Could you check a few things on this model? Use its own coordinates, in mm. A direction names the side the tool comes from. Give positions to 0.01 mm unless a question says otherwise; leave off trailing zeros. Loops run counter-clockwise (first coordinate to the right, second up) from the corner with the lowest first, then second, coordinate; pieces in that order, holes last.
1. Imagine slicing it at C-C (z = 11). List the corners of the cut face in (x, y) for me.
2. Imagine slicing it at B-B (x = 64.5). List the corners of the cut face in (y, z) for me (3 decimals), plus the area to 3 significant figures.
3. For faces 1 (the flat face through (-4, 5.334, 0)), 2 (the flat face through (47, -3.175, 0)), 3 (the cylindrical face through (8.82, 13.08, -2.9)), 4 (the flat face through (-1, 3.175, 22)), which set-ups out of +Z, -Z, +X, -X, +Y, -Y let a thin tool reach every point of the face, with its end or its side?
4. For P1, Ø4.5, axis at x = 59.5, z = 0, coming from the +Y side (3 decimals); P2, Ø6, axis at y = 13, z = -2.5, coming from the -X side; P3, Ø0.9, axis at y = -0.5, z = 22.5, coming from the -X side, each with a flat end and sliding along its axis, tell me the tip position at first contact or that it passes through.
5. I need wall thicknesses on line 1 along Y through (x, z) = (12.5, 0); line 2 along X through (y, z) = (0, -9); line 3 along Y through (x, z) = (41, 7) (3 decimals). Which ranges of each line are inside material? Lowest first, please.
6. Thinking about a two-plate mould opening in Z: for faces 5 (the cylindrical face through (-3.78, -0.07, 24.51)), 6 (the flat face through (47, 3.175, 0)), 7 (the cylindrical face through (-0.81, -0.07, 26.16)), which applies, +Z half, -Z half, draft (parallel to the pull), parting line (faces both ways), or undercut?
```python
from build123d import *

# Parameters (mm, degrees)
SKETCH2_W      = 12.192
SKETCH2_H      = 10.668
EXTRUDE1_DEPTH = 14.478
SKETCH3_W      = 14.224
SKETCH3_H      = 6.858
EXTRUDE2_DEPTH = 16.4592
EXTRUDE3_START = -1.651
EXTRUDE3_DEPTH = 1.651
FILLET1_R      = 3.175
SKETCH5_R      = 1.524
EXTRUDE4_DEPTH = 4.318
SKETCH6_W      = 15.24
SKETCH6_H      = 6.35
EXTRUDE5_DEPTH = 50.8


with BuildPart() as part:
    # Sketch1 → Revolve1 (revolve)
    with BuildSketch(Plane.XY, mode=Mode.PRIVATE) as revolve1_sk:
        Polygon((0, 13.3985), (17.399, 13.3985), (17.399, 11.938), (5.969, 11.938), (5.969, 0), (3.429, 0), (3.429, 11.938), (-6.731, 11.938), (-6.731, 17.272), (-1.651, 17.272), (-1.651, 18.923), (0, 18.923), align=None)
    revolve(revolve1_sk.sketch.rotate(Axis((-7.9375, 0, 0), (1, 0, 0)), 90), axis=Axis((-7.9375, 0, 0), (1, 0, 0)))

    # Sketch2 → Extrude1 (add)
    with BuildSketch(Plane.ZY.offset(-3.429)):
        Rectangle(SKETCH2_W, SKETCH2_H)
    extrude(amount=EXTRUDE1_DEPTH)

    # Sketch3 → Extrude2 (add)
    with BuildSketch(Plane(origin=(5.969, 0, 0), x_dir=(0, 0, -1), z_dir=(1, 0, 0))):
        Rectangle(SKETCH3_W, SKETCH3_H)
    extrude(amount=EXTRUDE2_DEPTH)

    # Sketch4 → Extrude3 (add)
    with BuildSketch(Plane.ZY.offset(1.651).offset(EXTRUDE3_START)):
        with BuildLine():
            Line((22.987, 3.175), (18.654739451, 3.175))
            ThreePointArc((18.654739451, 3.175), (18.923, 0), (18.654739451, -3.175))
            Line((18.654739451, -3.175), (22.987, -3.175))
            ThreePointArc((22.987, -3.175), (26.162, 0), (22.987, 3.175))
        make_face()
    extrude(amount=EXTRUDE3_DEPTH)

    # Fillet1
    fillet1_edges = [part.edges().sort_by_distance(p)[0] for p in [
        (-0.8255, 3.175, 18.654739451),
        (-0.8255, -3.175, 18.654739451),
    ]]
    fillet(fillet1_edges, radius=FILLET1_R)

    # Sketch5 → Extrude4 (add)
    with BuildSketch(Plane.ZY.offset(1.651)):
        with Locations(Location((22.987, 0, 0), (0, 0, 180))):
            Circle(SKETCH5_R)
    extrude(amount=EXTRUDE4_DEPTH)

    # Sketch6 → Extrude5 (add)
    with BuildSketch(Plane(origin=(22.4282, 0, 0), x_dir=(0, 0, -1), z_dir=(1, 0, 0))):
        Rectangle(SKETCH6_W, SKETCH6_H)
    extrude(amount=EXTRUDE5_DEPTH)


solid = part.part
```
Derived:
1. outline: (-6.73, -13.32) - (-1.65, -13.32) - (-1.65, -15.4) - (0, -15.4) - (0, -7.65) - (17.4, -7.65) - (17.4, -4.64) - (5.97, -4.64) - (5.97, 4.64) - (17.4, 4.64) - (17.4, 7.65) - (0, 7.65) - (0, 15.4) - (-1.65, 15.4) - (-1.65, 13.32) - (-6.73, 13.32) - (-6.73, 4.64) - (3.43, 4.64) - (3.43, -4.64) - (-6.73, -4.64) - close
2. outline: (-3.175, -7.62) - (3.175, -7.62) - (3.175, 7.62) - (-3.175, 7.62) - close
2. area: 96.8 mm2
3. face 1: -X
3. face 2: +Z, -Z, +X, -Y
3. face 3: +X
3. face 4: +Z, +X, -X, +Y
4. P1: stops at y = 3.175
4. P2: stops at x = -6.73
4. P3: stops at x = -5.97
5. line 1: y = -13.4 to -11.94, -3.43 to 3.43, 11.94 to 13.4
5. line 2: x = 3.43 to 5.97
5. line 3: y = -3.175 to 3.175
6. face 5: undercut
6. face 6: draft
6. face 7: +Z half
